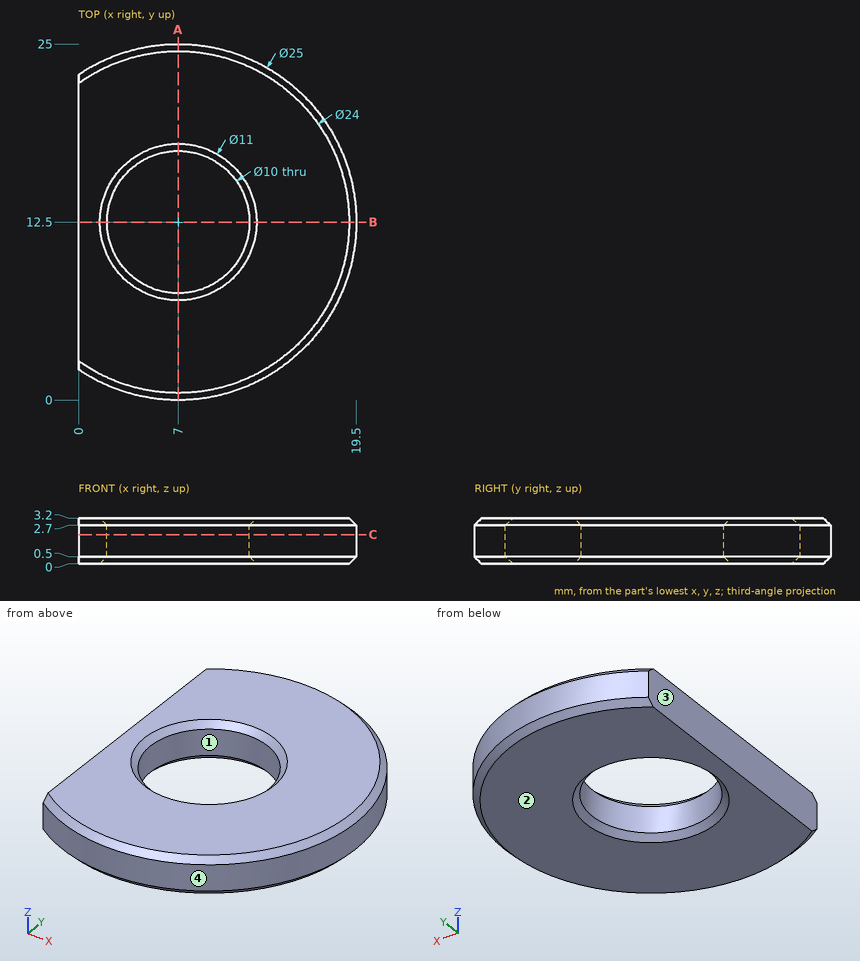
Input: dimensioned drawing with shaded views. Units: mm. Origin: part minimum x, y, z. Round coordinates to 2 decimals unless told otherwise and drop trailing zeros. Loops run counter-clockwise (first coordinate to the right, second up) from the corner with the lowest first, then second, coordinate; pieces in that order, holes last.
1) Section query A-A on x = 7. Return the cut outline in (y, z).
Ans:
outline: (0, 0.5) - (0.5, 0) - (7, 0) - (7.5, 0.5) - (7.5, 2.7) - (7, 3.2) - (0.5, 3.2) - (0, 2.7) - close; (17.5, 0.5) - (18, 0) - (24.5, 0) - (25, 0.5) - (25, 2.7) - (24.5, 3.2) - (18, 3.2) - (17.5, 2.7) - close
2) Pull-direction query (X, two-part tool) for the marked faces 1, 2, 3 and 4; classes: released by +X, released by -X, zero draft, split by the parting line, or undercut.
Ans:
face 1: undercut
face 2: zero draft
face 3: released by -X
face 4: split by the parting line
3) Material intervals for line 1 (Y direction, x = 7, z = 1.8); line 2 (Y direction, x = 10.5, z = 0.7); line 3 (X direction, y = 8.5, z = 0.1), sorted ascending.
Ans:
line 1: y = 0 to 7.5, 17.5 to 25
line 2: y = 0.5 to 8.93, 16.07 to 24.5
line 3: x = 0 to 3.37, 10.63 to 18.42
4) Section query C-C on z = 2.05. Return the cut outline in (x, y).
Ans:
outline: (0, 2.14) arc R12.5 ccw (long way) to (0, 22.86) - close; hole circle Ø10 at (7, 12.5)
5) Section query B-B on y = 12.5. Return the cut outline in (x, z).
Ans:
outline: (0, 0) - (1.5, 0) - (2, 0.5) - (2, 2.7) - (1.5, 3.2) - (0, 3.2) - close; (12, 0.5) - (12.5, 0) - (19, 0) - (19.5, 0.5) - (19.5, 2.7) - (19, 3.2) - (12.5, 3.2) - (12, 2.7) - close
6) Pin query (flat end, axial travel): pin 1 (1 mm diameter, centred on x = 3.5, z = 0.5, fed in from +Y); pin 2 (1 mm diameter, centred on y = 10, z = 3, fed in from +X); pin 3 (1 mm diameter, centred on y = 4, z = 3, fed in from +X). Return the tip coordinate at first contact, or that it passes through.
Ans:
pin 1: stops at y = 24.63
pin 2: stops at x = 19.32
pin 3: stops at x = 16.52
